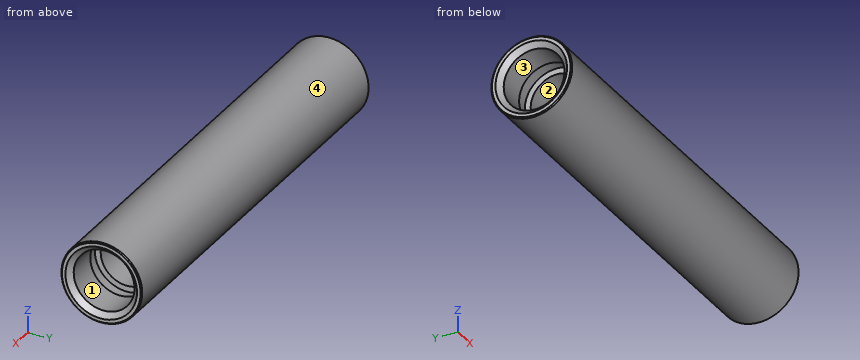
from build123d import *

# Parameters (mm, degrees)
F2_SIZE  = 0.5
F3_SIZE  = 2.5
F4_SIZE  = 2.5
F5_SIZE2 = 1.09999
F5_SIZE  = 0.99999
F6_SIZE2 = 1.06
F6_SIZE  = 1


# Not quite as in the source:
# - a fillet or chamfer is up to 0.001 mm smaller than in the source, because OpenCascade refuses the exact size


with BuildPart() as f1:
    # F0 (on Front) → F1 (revolve)
    with BuildSketch(Plane.XZ):
        Polygon((0, 18.8), (0, 14.15), (17, 14.15), (17, 15.25), (23, 15.25), (23, 12.5), (99.5, 12.5), (99.5, 18.8), align=None)
        Polygon((199, 18.8), (99.5, 18.8), (99.5, 12.5), (176, 12.5), (176, 15.25), (182, 15.25), (182, 14.15), (199, 14.15), align=None)
    revolve(axis=Axis((99.5, 0, 0), (-1, 0, 0)))

    # F2
    f2_edges = [f1.edges().sort_by_distance(p)[0] for p in [
        (199, 0, -18.8),
        (0, 0, -18.8),
    ]]
    chamfer(f2_edges, length=F2_SIZE)

    # F3
    f3_edges = [f1.edges().sort_by_distance(p)[0] for p in [
        (0, 0, -14.15),
    ]]
    chamfer(f3_edges, length=F3_SIZE)

    # F4
    f4_edges = [f1.edges().sort_by_distance(p)[0] for p in [
        (199, 0, -14.15),
    ]]
    chamfer(f4_edges, length=F4_SIZE)

    # F5 (size 1 and 1.1 in the source; OpenCascade refuses exactly that, so slightly less here)
    f5_edges = [f1.edges().sort_by_distance(p)[0] for p in [
        (17, 0, -14.15),
    ]]
    chamfer(f5_edges, length=F5_SIZE, length2=F5_SIZE2)

    # F6
    f6_edges = [f1.edges().sort_by_distance(p)[0] for p in [
        (182, 0, -15.25),
    ]]
    chamfer(f6_edges, length=F6_SIZE, length2=F6_SIZE2)


solid = f1.part
CAD build for the part. Positions are in the model's coordinates, mm. Face numbers are marked on the shaded views. A direction names the side the tool comes from. Give positions to 0.01 mm unless a question says otherwise; leave off trailing zeros. Loops run counter-clockwise (first coordinate to the right, second up) from the corner with the lowest first, then second, coordinate; pieces in that order, holes last. Notation, with made-up numbers: M 34,57 L 60,57 A28 cw 60,78 Z; hole C 29.25,-10 d9. An arc over 180 degrees is marked long. Answer in a Markdown table with one row per item. Add a question column.
Item 1: Drop flat-ended pins along their axis: P1, Ø5, axis at y = 8.5, z = -6, coming from the +X side; P2, Ø5, axis at x = 177, z = -7.5, coming from the -Y side; P3, Ø1.5, axis at y = 13.5, z = 0, coming from the -X side; P4, Ø22.5, axis at y = 6.5, z = 6.5, coming from the -X side. Give the stop position or say it passes through.
Item 2: Probe probe 1 along Y at (x, z) = (190, 0); probe 2 along Z at (x, y) = (32, 6); probe 3 along X at (y, z) = (9, -11). List the from-to ranges inside material, lowest first.
Item 3: Band-saw the part on A-A on x = 53.5. Give the cut face in (y, z).
Item 4: Mould opens along Z. For the marked faces 3 and 4 say: +Z half, -Z half, draft (parallel to the pull), parting line (faces both ways), or undercut.
Item 5: Tool access for the marked faces 1 and 2: list every direction of +Z, -Z, +X, -X, +Y, -Y with a clear straight run to the whole face (end or side of a thin tool).
Reply:
| question | item | result |
|---|---|---|
| 1 | P1 | stops at x = 176 |
| 1 | P2 | stops at y = -18.12 |
| 1 | P3 | stops at x = 2.4 |
| 1 | P4 | stops at x = 0 |
| 2 | probe 1 | y = -18.8 to -14.15, 14.15 to 18.8 |
| 2 | probe 2 | z = -17.82 to -10.97, 10.97 to 17.82 |
| 2 | probe 3 | x = 2.44 to 16.06, 23 to 176, 181.98 to 196.56 |
| 3 | outline | C 0,0 d37.6; hole C 0,0 d25 |
| 4 | face 3 | undercut |
| 4 | face 4 | parting line |
| 5 | face 1 | +X |
| 5 | face 2 | +X, -X |
